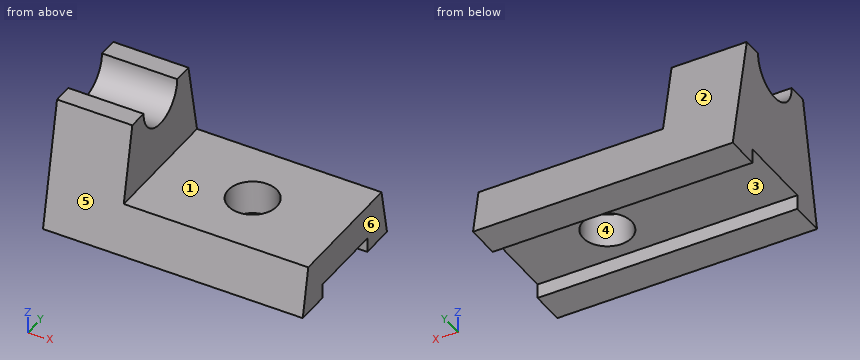
```python
from build123d import *

# Parameters (mm, degrees)
F1_DEPTH = 271.78
F2_W     = 193.04
F2_H     = 25.4
F2_H_2   = 20.32
F2_H_3   = 106.68
F3_DEPTH = 78.74
F4_R     = 25.4
F5_DEPTH = 76.2


with BuildPart() as f1:
    # F0 (on Right) → F1 (new body)
    with BuildSketch(Plane.YZ):
        with BuildLine():
            Line((-40.64, 0), (0, 0))
            Line((0, 0), (40.64, 0))
            Line((40.64, 0), (40.64, -15.24))
            Line((40.64, -15.24), (76.2, -15.24))
            Line((76.2, -15.24), (50.8, 114.3))
            Line((50.8, 114.3), (30.48, 114.3))
            ThreePointArc((30.48, 114.3), (0, 83.82), (-30.48, 114.3))
            Line((-30.48, 114.3), (-50.8, 114.3))
            Line((-50.8, 114.3), (-76.2, -15.24))
            Line((-76.2, -15.24), (-40.64, -15.24))
            Line((-40.64, -15.24), (-40.64, 0))
        make_face()
    extrude(amount=F1_DEPTH)

    # F2 (on face) → F3 (cut)
    with BuildSketch(Plane.XY.offset(114.3)):
        with Locations((175.26, 63.5)):
            Rectangle(F2_W, F2_H)
        with Locations((175.26, 40.64)):
            Rectangle(F2_W, F2_H_2)
        with Locations((175.26, -22.86)):
            Rectangle(F2_W, F2_H_3)
    extrude(amount=-F3_DEPTH, mode=Mode.SUBTRACT)

    # F4 (on face) → F5 (cut)
    with BuildSketch(Plane.XY.offset(35.56)):
        with Locations((175.26, 0)):
            Circle(F4_R)
    extrude(amount=-F5_DEPTH, mode=Mode.SUBTRACT)


solid = f1.part
```
The listing builds one solid part. Answer for the finished solid, in the listing's coordinates (mm). Face numbers are marked on the shaded views. A direction names the side the tool comes from. Give positions to 0.01 mm unless a question says otherwise; leave off trailing zeros. Loops run counter-clockwise (first coordinate to the right, second up) from the corner with the lowest first, then second, coordinate; pieces in that order, holes last. Notation, with made-up numbers: (41.25, -8.75) - (99.25, -8.75) arc R35 cw to (99.25, 23.25) - close; hole circle Ø11 at (40.5, 38). An arc over 180 degrees is marked (long way). Return JSON: item names as keys, results as strings. Group by question number.
1. Given pin 1 Ø4.5 at (x, z) = (72, -9) entering from +Y; pin 2 Ø3 at (x, y) = (84, 44) entering from +Z; pin 3 Ø7.5 at (x, z) = (123.5, -6.5) entering from -Y, each flat-ended and moving along its own axis, determine where each tip first touches the part or whether it passes through.
2. Straight lines are drawn through the part: line 1 (Z direction, x = 90.5, y = 50); line 2 (X direction, y = -56.5, z = 39); line 3 (Z direction, x = 245, y = -36.5). For each, find the intervals that lie inside material, in ascending order. Write a range as [from, to].
3. Find section D-D (x = 235). Write down the section's boundary in (y, z).
4. Find section B-B (y = 0). Write down the section's boundary in (x, z), then the cut area to 3 significant figures.
5. Find section A-A (x = 175.26). Write down the section's boundary in (y, z), then the cut area to 3 significant figures.
6. Find section C-C (z = 97). Write down the section's boundary in (x, y), then the cut area to 3 significant figures.
7. Which of the six approach directions +Z, -Z, +X, -X, +Y, -Y give full straight-line access (tool end or side, diameter ignored) to the marked faces 1, 2 and 3?
8. Determine the mould class of the marked faces 4, 5 and 6 for opening direction X: pulls with the +X half, pulls with the -X half, needs draft (parallel to the pull), parting line crosses it, or undercut.
Verdict:
{
 "1": {"pin 1": "stops at y = 75.42", "pin 2": "stops at z = 35.56", "pin 3": "stops at y = -75.22"},
 "2": {"line 1": "z = [-15.24, 35.56]", "line 2": "x = [0, 78.74]", "line 3": "z = [0, 35.56]"},
 "3": {"outline": "(-76.2, -15.24) - (-40.64, -15.24) - (-40.64, 0) - (40.64, 0) - (40.64, -15.24) - (76.2, -15.24) - (66.24, 35.56) - (-66.24, 35.56) - close"},
 "4": {"outline": "(0, 0) - (149.86, 0) - (149.86, 35.56) - (78.74, 35.56) - (78.74, 83.82) - (0, 83.82) - close; (200.66, 0) - (271.78, 0) - (271.78, 35.56) - (200.66, 35.56) - close", "area": "11,700 mm^2"},
 "5": {"outline": "(-76.2, -15.24) - (-40.64, -15.24) - (-40.64, 0) - (-25.4, 0) - (-25.4, 35.56) - (-66.24, 35.56) - close; (25.4, 0) - (40.64, 0) - (40.64, -15.24) - (76.2, -15.24) - (66.24, 35.56) - (25.4, 35.56) - close", "area": "4,190 mm^2"},
 "6": {"outline": "(0, -54.19) - (78.74, -54.19) - (78.74, -25.09) - (0, -25.09) - close; (0, 25.09) - (78.74, 25.09) - (78.74, 54.19) - (0, 54.19) - close", "area": "4,580 mm^2"},
 "7": {"face 1": "+Z, +X, +Y, -Y", "face 2": "+Z, +X, -X, +Y", "face 3": "-Z, +X, -X"},
 "8": {"face 4": "undercut", "face 5": "needs draft", "face 6": "pulls with the +X half"}
}
